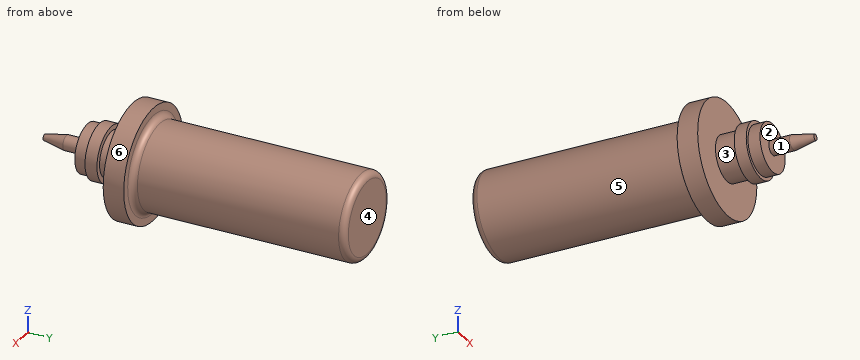
```python
from build123d import *

# Parameters (mm, degrees)
SKETCH1_R           = 10.00174333
BOSS_EXTRUDE3_DEPTH = 50
SKETCH4_R           = 13.27917762
BOSS_EXTRUDE4_DEPTH = 4.8
FILLET1_R           = 1.5
SKETCH5_R           = 5.290974817
BOSS_EXTRUDE5_DEPTH = 5
SKETCH6_R           = 6.466211651
BOSS_EXTRUDE6_DEPTH = 2.8
SKETCH7_R           = 5.659284008
BOSS_EXTRUDE7_DEPTH = 2.8
SKETCH8_R           = 1.715557864
BOSS_EXTRUDE8_DEPTH = 10
CHAMFER1_SIZE       = 1
CHAMFER1_SIZE2      = 5.144554016


with BuildPart() as part:
    # Sketch1 → Boss-Extrude3 (new body)
    with BuildSketch(Plane(origin=(0, 0, 0), x_dir=(1, 0, 0), z_dir=(0, 1, 0))):
        with Locations(Location((0, 0, 0), (0, 0, 270))):
            Circle(SKETCH1_R)
    extrude(amount=-BOSS_EXTRUDE3_DEPTH)

    # Sketch4 → Boss-Extrude4 (add)
    with BuildSketch(Plane.XZ.offset(50)):
        with Locations(Location((0, 0, 0), (0, 0, 270))):
            Circle(SKETCH4_R)
    extrude(amount=BOSS_EXTRUDE4_DEPTH)

    # Fillet1
    fillet1_edges = [part.edges().sort_by_distance(p)[0] for p in [
        (0, 0, -10.00174333),
        (0, -50, -10.00174333),
    ]]
    fillet(fillet1_edges, radius=FILLET1_R)

    # Sketch5 → Boss-Extrude5 (add)
    with BuildSketch(Plane(origin=(0, -54.8, 0), x_dir=(-1, 0, 0), z_dir=(0, -1, 0))):
        with Locations(Location((0, 0, 0), (0, 0, 90))):
            Circle(SKETCH5_R)
    extrude(amount=BOSS_EXTRUDE5_DEPTH)

    # Sketch6 → Boss-Extrude6 (add)
    with BuildSketch(Plane(origin=(0, -59.8, 0), x_dir=(-1, 0, 0), z_dir=(0, -1, 0))):
        with Locations(Location((0, 0, 0), (0, 0, 90))):
            Circle(SKETCH6_R)
    extrude(amount=BOSS_EXTRUDE6_DEPTH)

    # Sketch7 → Boss-Extrude7 (add)
    with BuildSketch(Plane(origin=(0, -62.6, 0), x_dir=(-1, 0, 0), z_dir=(0, -1, 0))):
        with Locations(Location((0, 0, 0), (0, 0, 90))):
            Circle(SKETCH7_R)
    extrude(amount=BOSS_EXTRUDE7_DEPTH)

    # Sketch8 → Boss-Extrude8 (add)
    with BuildSketch(Plane.XZ.offset(65.4)):
        with Locations(Location((0, 0, 0), (0, 0, 270))):
            Circle(SKETCH8_R)
    extrude(amount=BOSS_EXTRUDE8_DEPTH)

    # Chamfer1
    chamfer1_edges = [part.edges().sort_by_distance(p)[0] for p in [
        (0, -75.4, 1.715557864),
    ]]
    chamfer1_side = [part.faces().sort_by_distance(p)[0] for p in [
        (0, -75.4, 0),
    ]]
    chamfer(chamfer1_edges, length=CHAMFER1_SIZE, length2=CHAMFER1_SIZE2, reference=chamfer1_side[0])


solid = part.part
```
CAD build for the part. Positions are in the model's coordinates, mm. Face numbers are marked on the shaded views. A direction names the side the tool comes from. Round coordinates to 2 decimals unless told otherwise and drop trailing zeros. Write each loop counter-clockwise with the first axis right and the second up, starting at its lowest first coordinate (ties: lowest second). Pieces come first, ordered by that corner, then holes.
Item 1: Drop flat-ended pins along their axis: pin 1 Ø6 at (x, z) = (-8, 3.5) entering from -Y; pin 2 Ø6 at (y, z) = (-66, 8) entering from -X; pin 3 Ø8 at (y, z) = (-20.5, 2.5) entering from +X. Give the stop position or say it passes through.
Filled in:
pin 1: stops at y = -62.6
pin 2: stops at x = -2.53
pin 3: stops at x = 10
Item 2: Mould opens along Y. For the marked faces 1, 2, 3 and 4 say: released by +Y, released by -Y, zero draft, split by the parting line, or undercut.
Filled in:
face 1: zero draft
face 2: released by -Y
face 3: undercut
face 4: released by +Y
Item 3: Drill centre lines: L1, parallel to Y at x = -4, z = 7.5; L2, parallel to Y at x = 12, z = 1.25; L3, parallel to Z at x = 6.5, y = -19. Where is each one in solid material? Low to high.
Filled in:
L1: y = -54.8 to 0
L2: y = -54.8 to -50
L3: z = -7.6 to 7.6
Item 4: Band-saw the part on C-C on y = -41. Write the cut outline in (x, z).
Filled in:
outline: circle Ø20 at (0, 0)
Item 5: Tool access for the marked faces 5 and 6: list every direction of +Z, -Z, +X, -X, +Y, -Y with a clear straight run to the whole face (end or side of a thin tool).
Filled in:
face 5: +Y
face 6: +Y, -Y
